Geometry check sheet. Reference: drawing and pictorial views, mm from the part's lowest x, y, z. Give positions to 0.01 mm unless a question says otherwise; leave off trailing zeros. Write each loop counter-clockwise with the first axis right and the second up, starting at its lowest first coordinate (ties: lowest second). Pieces come first, ordered by that corner, then holes. Notation, with made-up numbers: (-22.75, -27.5) - (-11.75, -27.5) arc R18 ccw to (-11.75, -9.5) - close; hole circle Ø10 at (21, 71). An arc over 180 degrees is marked (long way). Write item = value, one per line. Start each with the question number.
(1) Section check A-A, the plane y = 28. Enter the section's corners in (x, z).
(2) Draft check along Y on the marked faces 1, 2 and 3. Enter one of: pulls with the +Y half, pulls with the -Y half, needs draft (parallel to the pull), parting line crosses it, or undercut.
(3) Depth check by flat-ended pin: pin 1 Ø1 at (x, z) = (3.5, 7) entering from +Y; pin 2 Ø1 at (x, z) = (2.5, 5.5) entering from -Y; pin 3 Ø11 at (x, y) = (28, 28) entering from +Z (3 decimals); pin 4 Ø2 at (y, z) = (3, 6.5) entering from +X. Enter the tip coordinate at first touch or a pass-through.
(4) Thickness scan on L1, parallel to Y at x = 28, z = 4; L2, parallel to X at y = 30, z = 10; L3, parallel to Y at x = 32, z = 0.5. Record the ranges inside material, lowest first.
(5) Section check B-B, the plane z = 8.75. Enter the section's corners in (x, y), plus the area to 3 significant figures.
(6) Section check D-D, the plane x = 50.5. Enter the section's corners in (y, z), plus the area to 3 significant figures.
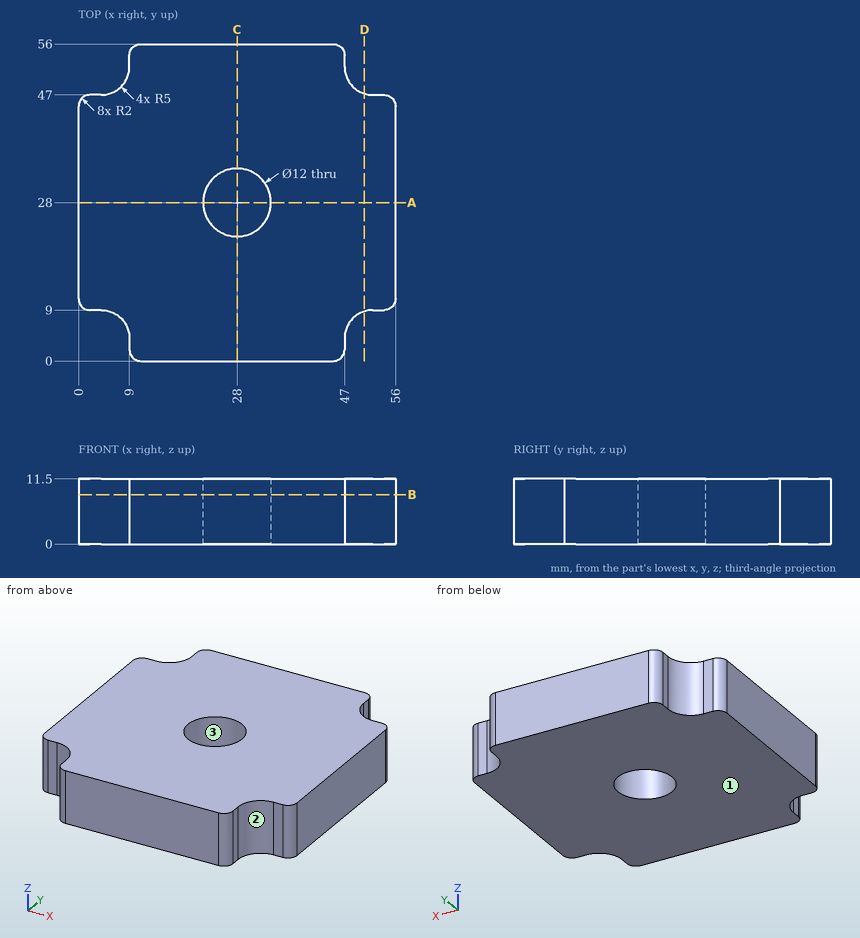
Model answer:
q1.outline = (0, 0) - (22, 0) - (22, 11.5) - (0, 11.5) - close; (34, 0) - (56, 0) - (56, 11.5) - (34, 11.5) - close
q2.face_1 = needs draft
q2.face_2 = pulls with the -Y half
q2.face_3 = undercut
q3.pin_1 = 47
q3.pin_2 = 9
q3.pin_3 = through
q3.pin_4 = 47
q4.L1 = 0 to 22, 34 to 56
q4.L2 = 0 to 22.34, 33.66 to 56
q4.L3 = 0 to 23.53, 32.47 to 56
q5.outline = (0, 11) arc R2 ccw to (2, 9) - (4, 9) arc R5 cw to (9, 4) - (9, 2) arc R2 ccw to (11, 0) - (45, 0) arc R2 ccw to (47, 2) - (47, 4) arc R5 cw to (52, 9) - (54, 9) arc R2 ccw to (56, 11) - (56, 45) arc R2 ccw to (54, 47) - (52, 47) arc R5 cw to (47, 52) - (47, 54) arc R2 ccw to (45, 56) - (11, 56) arc R2 ccw to (9, 54) - (9, 52) arc R5 cw to (4, 47) - (2, 47) arc R2 ccw to (0, 45) - close; hole circle Ø12 at (28, 28)
q5.area = 2,710 mm²
q6.outline = (8.77, 0) - (47.23, 0) - (47.23, 11.5) - (8.77, 11.5) - close
q6.area = 442 mm²
